Source: CAD feature listing. Evaluate the final solid. Frame: model axes, mm. A direction names the side the tool comes from. Coordinates: 2 decimals unless noted, no trailing zeros. Order: outer loops, then holes, each group sorted by start corner. A loop starts at its lowest first (then second) coordinate and runs counter-clockwise, first axis right, second up. Notation, with made-up numbers: (-21, 48) - (18, 48) arc R37 cw to (18, 84) - close; hole circle Ø9 at (30, -24). An arc over 180 degrees is marked (long way). One line per question, with ' | ' between items.
from build123d import *

# Parameters (mm, degrees)
BOSS_EXTRUDE1_DEPTH      = 306.3875
BOSS_EXTRUDE1_2_DEPTH    = 306.3875
BOSS_EXTRUDE1_3_DEPTH    = 306.3875
SKETCH3_W                = 120.65
SKETCH3_H                = 19.685
BOSS_EXTRUDE1_4_DEPTH    = 306.3875
LPATTERN1_COUNT          = 3
LPATTERN1_PITCH          = 244.475
BOSS_EXTRUDE2_DEPTH      = 304.8
SKETCH5_W                = 606.679
SKETCH5_H                = 2.54
BOSS_EXTRUDE3_DEPTH      = 609.6
BOSS_EXTRUDE4_DEPTH      = 285.75
BOSS_EXTRUDE4_DEPTH_BACK = 285.75


with BuildPart() as part:
    # Sketch3 → Boss-Extrude1 (new, symmetric)
    with BuildSketch(Plane.XY):
        Polygon((-304.8, -76.2), (-304.8, -73.025), (-287.655, -55.5625), (-201.295, -55.5625), (-184.15, -73.025), (-184.15, -76.2), align=None)
    extrude(amount=BOSS_EXTRUDE1_DEPTH, both=True)



with BuildPart() as body_2:
    # Sketch3 → Boss-Extrude1 2 (new, symmetric)
    with BuildSketch(Plane.XY):
        Polygon((184.15, -73.025), (184.15, -76.2), (304.8, -76.2), (304.8, -73.025), (287.655, -55.5625), (201.295, -55.5625), align=None)
    extrude(amount=BOSS_EXTRUDE1_2_DEPTH, both=True)


with BuildPart() as body_3:
    # Sketch3 → Boss-Extrude1 3 (new, symmetric)
    with BuildSketch(Plane.XY):
        Polygon((-60.325, -76.2), (60.325, -76.2), (60.325, -73.025), (43.18, -55.5625), (-43.18, -55.5625), (-60.325, -73.025), align=None)
    extrude(amount=BOSS_EXTRUDE1_3_DEPTH, both=True)


with BuildPart() as body_4:
    # Sketch3 → Boss-Extrude1 4 (new, symmetric)
    with BuildSketch(Plane.XY):
        with Locations((-244.475, 63.8175)):
            Rectangle(SKETCH3_W, SKETCH3_H)
    extrude(amount=BOSS_EXTRUDE1_4_DEPTH, both=True)


with BuildPart() as lpattern1_1:
    # LPattern1: pattern copy
    add(body_4.part.moved(Location(Vector(1, 0, 0) * (1 * LPATTERN1_PITCH))))


with BuildPart() as lpattern1_2:
    # LPattern1: pattern copy
    add(body_4.part.moved(Location(Vector(1, 0, 0) * (2 * LPATTERN1_PITCH))))


with BuildPart() as part_1:
    add(part.part)

    add(body_2.part)  # Boss-Extrude2 merges body 2

    add(body_3.part)  # Boss-Extrude2 merges body 3

    add(body_4.part)  # Boss-Extrude2 merges body 4

    add(lpattern1_1.part)  # Boss-Extrude2 merges LPattern1_1

    add(lpattern1_2.part)  # Boss-Extrude2 merges LPattern1_2
    # Sketch4 → Boss-Extrude2 (add, symmetric)
    with BuildSketch(Plane(origin=(0, 0, 0), x_dir=(0, 0, -1), z_dir=(1, 0, 0))):
        Polygon((-306.3875, 76.2), (-306.3875, 50.927), (-282.448, 50.927), (-282.448, -52.5145), (-306.3875, -52.5145), (-306.3875, -76.2), (-303.3395, -76.2), (-303.3395, -55.5625), (-279.4, -55.5625), (-279.4, 53.975), (-303.3395, 53.975), (-303.3395, 76.2), align=None)
        Polygon((303.3395, 53.975), (303.3395, 76.2), (306.3875, 76.2), (306.3875, 50.927), (282.448, 50.927), (282.448, -52.5145), (306.3875, -52.5145), (306.3875, -76.2), (303.3395, -76.2), (303.3395, -55.5625), (279.4, -55.5625), (279.4, 53.975), align=None)
    extrude(amount=BOSS_EXTRUDE2_DEPTH, both=True)

    # Sketch5 → Boss-Extrude3 (add)
    with BuildSketch(Plane(origin=(304.8, 0, 0), x_dir=(0, 0, -1), z_dir=(1, 0, 0))):
        with Locations((0, 74.93)):
            Rectangle(SKETCH5_W, SKETCH5_H)
    extrude(amount=-BOSS_EXTRUDE3_DEPTH)

    # Sketch6 → Boss-Extrude4 (add, two sides: drawn at the far end of the back side and taken through both)
    with BuildSketch(Plane(origin=(0, 0, 0), x_dir=(0, 0, -1), z_dir=(1, 0, 0)).offset(-BOSS_EXTRUDE4_DEPTH_BACK)):
        with BuildLine():
            Line((-17.4625, 53.975), (-17.4625, -55.5625))
            Line((-17.4625, -55.5625), (17.4625, -55.5625))
            ThreePointArc((17.4625, -55.5625), (14.672692091, -48.827307909), (7.9375, -46.0375))
            Line((7.9375, -46.0375), (-7.9375, -46.0375))
            Line((-7.9375, -46.0375), (-7.9375, 44.45))
            Line((-7.9375, 44.45), (7.9375, 44.45))
            ThreePointArc((7.9375, 44.45), (14.672692091, 47.239807909), (17.4625, 53.975))
            Line((17.4625, 53.975), (-17.4625, 53.975))
        make_face()
    extrude(amount=BOSS_EXTRUDE4_DEPTH + BOSS_EXTRUDE4_DEPTH_BACK)


solid = part_1.part
(1) Set-up query: faces 3 (the flat face through (-4, 0, 282.448)), 4 (the flat face through (121, 53.975, 0)), 5 (the flat face through (300, -61, -303.34)), 6 (the flat face through (-4, -46.038, 0)). Return all of +Z, -Z, +X, -X, +Y, -Y with unobstructed straight access to the full face (end or side cutting, diameter ignored); none if empty.
Taken from the geometry:
face 3: +Z, +X, -X | face 4: none | face 5: +X | face 6: +X, -X
(2) Cut plane A-A (y = 30). Return the cut outline in (x, z).
Taken from the geometry:
outline: (-304.8, -282.45) - (304.8, -282.45) - (304.8, -279.4) - (-304.8, -279.4) - close; (-304.8, 279.4) - (304.8, 279.4) - (304.8, 282.45) - (-304.8, 282.45) - close; (-285.75, 7.94) - (285.75, 7.94) - (285.75, 17.46) - (-285.75, 17.46) - close
(3) Cut plane B-B (z = -119.5). State how many separate pieces and enclosed holes the cut face has, and give its area (3 significant figures).
Taken from the geometry:
separate pieces: 4 | enclosed holes: 0 | area: 15,200 mm²
(4) Pin query (flat end, axial travel): P1, Ø2, axis at x = -156.5, y = 42, coming from the -Z side. Return the tip coordinate at first contact, or that it passes through.
Taken from the geometry:
P1: stops at z = -282.45
(5) Material intervals for L1, parallel to Z at x = 246, y = -2; L2, parallel to X at y = 68, z = 91.5 (3 decimals); L3, parallel to Y at x = 214.5, z = -144.5 (1 decimal), sorted ascending. Write a range as from..to.
Taken from the geometry:
L1: z = -282.45..-279.4, 7.94..17.46, 279.4..282.45 | L2: x = -304.8..-184.15, -60.325..60.325, 184.15..304.8 | L3: y = -76.2..-55.6, 54..76.2
(6) Pull-direction query (Y, two-part tool) for faces 1 (the flat face through (-4, 0, 17.462)), 2 (the flat face through (4, -64, -306.388)); classes: pulls with the +Y half, pulls with the -Y half, needs draft (parallel to the pull), parting line crosses it, or undercut.
Taken from the geometry:
face 1: undercut | face 2: needs draft
